Autodesk Inventor part; units mm, degrees
ref_plane "YZ Plane" through (0, 0, 0) normal (1, 0, 0) x (0, 1, 0)
ref_plane "XZ Plane" through (0, 0, 0) normal (0, 1, 0) x (-1, 0, 0)
ref_plane "XY Plane" through (0, 0, 0) normal (0, 0, 1) x (1, 0, 0)
sketch "Sketch9" plane through (0, 0, 0) normal (0, 1, 0) x (-1, 0, 0)
  line L0 (15, 15) -> (-15, 15)
  line L1 (-15, 15) -> (-15, -15)
  line L2 (-15, -15) -> (15, -15)
  line L3 (15, -15) -> (15, 15)
  line L4 (15, 15) -> (-15, -15) construction
  line L5 (-15, 15) -> (15, -15) construction
  line L6 (-13, 13) -> (13, 13)
  line L7 (13, 13) -> (13, -13)
  line L8 (13, -13) -> (-13, -13)
  line L9 (-13, -13) -> (-13, 13)
  point P0 (0, 0)
  dimension "d172" = 30
  dimension "d173" = 30
  dimension "d174" = 2
extrude "Extrusion3" add sketch "Sketch9" against normal blind 420
sketch "Sketch10" plane through (0, 0, 0) normal (1, 0, 0) x (0, 1, 0)
  line L0 (0, 15) -> (0, -15) construction
  line L1 (0, 15) -> (-420, 15) construction
  line L2 (-420, -15) -> (-420, 15) construction
  line L3 (0, -15) -> (-420, -15) construction
  line L4 (-68.5, 8.5) -> (-51.5, 8.5)
  line L5 (-51.5, 8.5) -> (-51.5, -8.5)
  line L6 (-51.5, -8.5) -> (-68.5, -8.5)
  line L7 (-68.5, -8.5) -> (-68.5, 8.5)
  line L8 (-68.5, 8.5) -> (-51.5, -8.5) construction
  line L9 (-51.5, 8.5) -> (-68.5, -8.5) construction
  line L10 (-238.5, 8.5) -> (-221.5, 8.5)
  line L11 (-221.5, 8.5) -> (-221.5, -8.5)
  line L12 (-221.5, -8.5) -> (-238.5, -8.5)
  line L13 (-238.5, -8.5) -> (-238.5, 8.5)
  line L14 (-238.5, 8.5) -> (-221.5, -8.5) construction
  line L15 (-221.5, 8.5) -> (-238.5, -8.5) construction
  line L16 (-413.5, 8.5) -> (-396.5, 8.5)
  line L17 (-396.5, 8.5) -> (-396.5, -8.5)
  line L18 (-396.5, -8.5) -> (-413.5, -8.5)
  line L19 (-413.5, -8.5) -> (-413.5, 8.5)
  line L20 (-413.5, 8.5) -> (-396.5, -8.5) construction
  line L21 (-396.5, 8.5) -> (-413.5, -8.5) construction
  circle A0 centre (-470, 0) radius 8.5
  line L22 (0, 0) -> (30, 0)
  circle A1 centre (-60, 0) radius 8.5
  circle A2 centre (-230, 0) radius 8.5
  circle A3 centre (-405, 0) radius 8.5
  dimension "d177" = 17
  dimension "d178" = 17
  dimension "d181" = 30
  dimension "d182" = 90
  dimension "d183" = 260
  dimension "d184" = 435
  dimension "d185" = 500
  dimension "d186" = 17
extrude "Extrusion4" cut sketch "Sketch10" along normal through all contours A1 | A2 | A3
properties part number "TZS 1752 FDS 1200 way tube 2" material "Stainless Steel"
Geometry: final body of the model. Coordinates: model frame, mm. A direction names the side the tool comes from. Give positions to 0.01 mm unless a question says otherwise; leave off trailing zeros. Write each loop counter-clockwise with the first axis right and the second up, starting at its lowest first coordinate (ties: lowest second). Pieces come first, ordered by that corner, then holes.
(1) Cut plane B-B, the plane y = -41. Return loops of the section in (x, z).
(2) Cut plane D-D, the plane y = -405. Return loops of the section in (x, z), then the cut area to 3 significant figures.
(3) Cut plane A-A, the plane x = 1.5. Return loops of the section in (y, z), then the cut area to 3 significant figures.
(4) First-contact query: P1, Ø10, axis at x = -6.5, z = 1.5, coming from the -Y side; P2, Ø13.5, axis at y = -405, z = 0, coming from the +X side. Flat tips, straight axial feed; report the tip coordinate or a pass-through.
(5) Mould query, pull axis X, two halves, no side actions, for faces 4 (the flat face through (-15, -207, 0)), 5 (the flat face through (14, 0, 0)), 6 (the flat face through (13, -207, 0)). Classes: released by +X, released by -X, zero draft, split by the parting line, or undercut.
(6) Access query for faces 1 (the cylindrical face through (13.99, -413.49, -0.37)), 2 (the flat face through (0, -207, 13)), 3 (the flat face through (15, -207, 0)). Directions: +Z, -Z, +X, -X, +Y, -Y. A direction counts if a zero-diameter tool reaches every point of the face in a straight line with its end or side. Return the directions, or none.
(7) Ray query, line 1 (Y direction, x = 13.6, z = 0); line 2 (Z direction, x = 14.15, y = -405); line 3 (Z direction, x = 4.5, y = -138). Return the intervals inside material, ascending.
(8) Cut plane C-C, the plane z = 0. Return loops of the section in (x, y).
Values follow:
1. outline: (-15, -15) - (15, -15) - (15, 15) - (-15, 15) - close; hole (-13, -13) - (13, -13) - (13, 13) - (-13, 13) - close
2. outline: (-15, -15) - (15, -15) - (15, -8.5) - (13, -8.5) - (13, -13) - (-13, -13) - (-13, 13) - (13, 13) - (13, 8.5) - (15, 8.5) - (15, 15) - (-15, 15) - close
2. area: 190 mm2
3. outline: (-420, -15) - (0, -15) - (0, -13) - (-420, -13) - close; (-420, 13) - (0, 13) - (0, 15) - (-420, 15) - close
3. area: 1,680 mm2
4. P1: passes through
4. P2: stops at x = -13
5. face 4: released by -X
5. face 5: zero draft
5. face 6: undercut
6. face 1: +X
6. face 2: +Y, -Y
6. face 3: +Z, -Z, +X, +Y, -Y
7. line 1: y = -420 to -413.5, -396.5 to -238.5, -221.5 to -68.5, -51.5 to 0
7. line 2: z = -15 to -8.5, 8.5 to 15
7. line 3: z = -15 to -13, 13 to 15
8. outline: (-15, -420) - (-13, -420) - (-13, 0) - (-15, 0) - close; (13, -420) - (15, -420) - (15, -413.5) - (13, -413.5) - close; (13, -396.5) - (15, -396.5) - (15, -238.5) - (13, -238.5) - close; (13, -221.5) - (15, -221.5) - (15, -68.5) - (13, -68.5) - close; (13, -51.5) - (15, -51.5) - (15, 0) - (13, 0) - close
